from build123d import *

# Parameters (mm, degrees)
F0_R     = 20
F1_DEPTH = 30


with BuildPart() as f1:
    # F0 (on Front) → F1 (new body)
    with BuildSketch(Plane.XZ):
        with BuildLine():
            Line((-11.634756, 26.593659), (-65.40378, 49.217329))
            ThreePointArc((-65.40378, 49.217329), (-77.942286, 45), (-75.325348, 32.032671))
            Line((-75.325348, 32.032671), (-28.848162, -3.220835))
            ThreePointArc((-28.848162, -3.220835), (-20.997346, -12.122824), (-17.213406, -23.372824))
            Line((-17.213406, -23.372824), (-9.921567, -81.25))
            ThreePointArc((-9.921567, -81.25), (0, -90), (9.921567, -81.25))
            Line((9.921567, -81.25), (17.213406, -23.372824))
            ThreePointArc((17.213406, -23.372824), (20.997346, -12.122824), (28.848162, -3.220835))
            Line((28.848162, -3.220835), (75.325348, 32.032671))
            ThreePointArc((75.325348, 32.032671), (77.942286, 45), (65.40378, 49.217329))
            Line((65.40378, 49.217329), (11.634756, 26.593659))
            ThreePointArc((11.634756, 26.593659), (0, 24.245647), (-11.634756, 26.593659))
        make_face()
        with BuildLine():
            ThreePointArc((5, -80), (0, -85), (-5, -80))
            Line((-5, -80), (-5, -40))
            ThreePointArc((-5, -40), (0, -35), (5, -40))
            Line((5, -40), (5, -80))
        make_face(mode=Mode.SUBTRACT)
        with BuildLine():
            ThreePointArc((-71.782032, 35.669873), (-73.612159, 42.5), (-66.782032, 44.330127))
            Line((-66.782032, 44.330127), (-32.141016, 24.330127))
            ThreePointArc((-32.141016, 24.330127), (-30.310889, 17.5), (-37.141016, 15.669873))
            Line((-37.141016, 15.669873), (-71.782032, 35.669873))
        make_face(mode=Mode.SUBTRACT)
        Circle(F0_R, mode=Mode.SUBTRACT)
        with BuildLine():
            ThreePointArc((66.782032, 44.330127), (73.612159, 42.5), (71.782032, 35.669873))
            Line((71.782032, 35.669873), (37.141016, 15.669873))
            ThreePointArc((37.141016, 15.669873), (30.310889, 17.5), (32.141016, 24.330127))
            Line((32.141016, 24.330127), (66.782032, 44.330127))
        make_face(mode=Mode.SUBTRACT)
    extrude(amount=F1_DEPTH)


solid = f1.part
Design review of the part built by this model. Coordinates are the model's own, in mm. A direction names the side the tool comes from. Coordinates: 2 decimals unless noted, no trailing zeros. Loops run counter-clockwise (first coordinate to the right, second up) from the corner with the lowest first, then second, coordinate; pieces in that order, holes last. Notation, with made-up numbers: (37, 18) -> (57, 18) arc R23 ccw to (57, 38) -> close; hole circle Ø3 at (79, -40). An arc over 180 degrees is marked (long way). Use a Markdown table: item, result. Add a question column.
Item 1: Machinability: for faces 1 (the flat face through (-5, -15, -60)), 2 (the flat face through (-38.143, -14.79, 37.747)), 3 (the flat face through (-6, 0, -20)), which of the approach directions +Z, -Z, +X, -X, +Y, -Y give a long, thin tool a straight path to every point of the face, cutting with its end or side? Answer none if there is none.
Item 2: Wall thickness on L1, parallel to Z at x = 0, y = -22; L2, parallel to X at y = -17, z = 27; L3, parallel to X at y = -21.75, z = 41: over which ranges is each line inside the solid? List them lowest first. Write a range as from..to.
Item 3: We need section D-D, the plane y = -14. Write out the cut boundary in (x, z).
Item 4: Clearance check with flat-ended pins moving along their axes: P1, Ø1, axis at y = -26, z = -18.5, coming from the +X side; P2, Ø15, axis at y = -13.5, z = -66, coming from the -X side; P3, Ø15, axis at y = -11.5, z = -60, coming from the +X side. State where each tip first meets the part, or that it passes through.
Item 5: We need section A-A, the plane x = 0. Write out the cut boundary in (y, z), and give its area (3 significant figures).
Item 6: We need section C-C, the plane x = -41. Write out the cut boundary in (y, z), and give its area (3 significant figures).
Item 7: The part is to be moulded in two halves that separate along X. For faces 4 (the flat face through (54.704, -14.79, 25.81)), 5 (the cylindrical face through (-21.08, -14.79, -11.98)), 6 (the flat face through (51.76, -14.79, 14.16)), say which applies: +X half, -X half, draft (parallel to the pull), parting line (faces both ways), or undercut.
Item 8: We need section B-B, the plane z = 0. Write out the cut boundary in (x, y).
Numbers:
| question | item | result |
|---|---|---|
| 1 | face 1 | +Y, -Y |
| 1 | face 2 | +Z, +Y, -Y |
| 1 | face 3 | +Z, -Z, +X, -X, +Y |
| 2 | L1 | z = -90..-85, -35..-20, 20..24.25 |
| 2 | L2 | x = -68.69..-56.77, -36.77..-12.6, 12.6..36.77, 56.77..68.69 |
| 2 | L3 | x = -79.23..-74.18, -61.01..-45.87, 45.87..61.01, 74.18..79.23 |
| 3 | outline | (-75.33, 32.03) -> (-28.85, -3.22) arc R30 cw to (-17.21, -23.37) -> (-9.92, -81.25) arc R10 ccw to (9.92, -81.25) -> (17.21, -23.37) arc R30 cw to (28.85, -3.22) -> (75.33, 32.03) arc R10 ccw to (65.4, 49.22) -> (11.63, 26.59) arc R30 cw to (-11.63, 26.59) -> (-65.4, 49.22) arc R10 ccw to start; hole (-71.78, 35.67) -> (-37.14, 15.67) arc R5 ccw to (-32.14, 24.33) -> (-66.78, 44.33) arc R5 ccw to start; hole circle Ø40 at (0, 0); hole (-5, -80) arc R5 ccw to (5, -80) -> (5, -40) arc R5 ccw to (-5, -40) -> close; hole (32.14, 24.33) arc R5 ccw to (37.14, 15.67) -> (71.78, 35.67) arc R5 ccw to (66.78, 44.33) -> close |
| 4 | P1 | stops at x = 18.4 |
| 4 | P2 | stops at x = -12.79 |
| 4 | P3 | stops at x = 13.54 |
| 5 | outline | (-30, -90) -> (0, -90) -> (0, -85) -> (-30, -85) -> close; (-30, -35) -> (0, -35) -> (0, -20) -> (-30, -20) -> close; (-30, 20) -> (0, 20) -> (0, 24.25) -> (-30, 24.25) -> close |
| 5 | area | 727 mm^2 |
| 6 | outline | (-30, 6) -> (0, 6) -> (0, 17.9) -> (-30, 17.9) -> close; (-30, 29.44) -> (0, 29.44) -> (0, 38.95) -> (-30, 38.95) -> close |
| 6 | area | 642 mm^2 |
| 7 | face 4 | undercut |
| 7 | face 5 | -X half |
| 7 | face 6 | +X half |
| 8 | outline | (-33.09, -30) -> (-20, -30) -> (-20, 0) -> (-33.09, 0) -> close; (20, -30) -> (33.09, -30) -> (33.09, 0) -> (20, 0) -> close |
